Build history of the part. All positions in model axes, mm. Face numbers are marked on the shaded views. A direction names the side the tool comes from. Round coordinates to 2 decimals unless told otherwise and drop trailing zeros. Loops run counter-clockwise (first coordinate to the right, second up) from the corner with the lowest first, then second, coordinate; pieces in that order, holes last. Notation, with made-up numbers: M -35,26.5 L 20,26.5 A19 ccw 20,47.5 Z; hole C 51.5,16.25 d4. An arc over 180 degrees is marked long. Write each question's results on one line, items separated by ' | '. Start each with the question number.
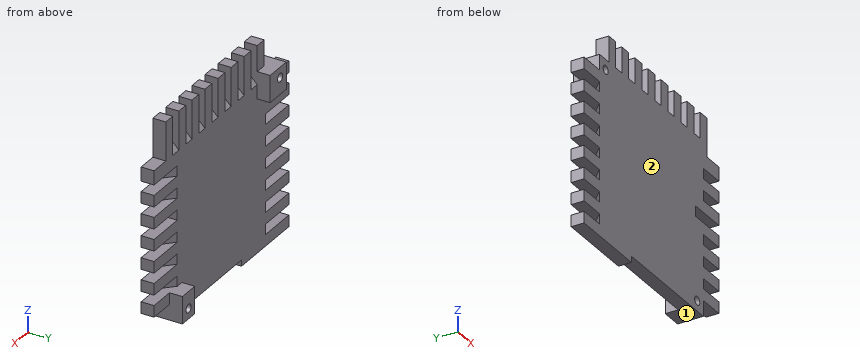
```python
from build123d import *

# Parameters (mm, degrees)
BASE_OUTLINE_R      = 0.5
BOSS_EXTRUDE1_DEPTH = 1.5
DRAFT2_ANGLE        = 45
SPACER_OUTLINE_W    = 3.14
SPACER_OUTLINE_H    = 3.14
SPACER_OUTLINE_W_2  = 2.4
SPACER_OUTLINE_H_2  = 3.16
BOSS_EXTRUDE2_DEPTH = 1.5
SKETCH1_3_R         = 0.5
CUT_EXTRUDE1_DEPTH  = 5.5


with BuildPart() as part:
    # Base outline → Boss-Extrude1 (new body)
    with BuildSketch(Plane(origin=(0, 0, 0), x_dir=(1, 0, 0), z_dir=(0, 1, 0))):
        Polygon((6.201628494, 20.2), (20.2, 20.2), (20.2, 18.38), (23.2, 18.38), (23.2, 17.04), (20.2, 17.04), (18.7, 17.04), (18.7, 15.84), (20.2, 15.84), (23.2, 15.84), (23.2, 14.5), (20.2, 14.5), (18.7, 14.5), (18.7, 13.3), (20.2, 13.3), (23.2, 13.3), (23.2, 11.96), (20.2, 11.96), (18.7, 11.96), (18.7, 10.76), (20.2, 10.76), (23.2, 10.76), (23.2, 9.42), (20.2, 9.42), (18.7, 9.42), (18.7, 8.22), (20.2, 8.22), (23.2, 8.22), (23.2, 6.88), (20.2, 6.88), (18.7, 6.88), (18.7, 5.68), (20.2, 5.68), (23.2, 5.68), (23.2, 4.34), (20.2, 4.34), (18.7, 4.34), (18.7, 3.14), (20.2, 3.14), (23.2, 3.14), (23.2, 1.5), (20.92, 1.5), (20.92, -3), (19.58, -3), (19.58, 0), (19.58, 1.5), (18.38, 1.5), (18.38, 0), (18.38, -3), (17.04, -3), (17.04, 0), (17.04, 1.5), (15.84, 1.5), (15.84, 0), (15.84, -3), (14.5, -3), (14.5, 0), (14.5, 1.5), (13.3, 1.5), (13.3, 0), (13.3, -3), (11.96, -3), (11.96, 0), (11.96, 1.5), (10.76, 1.5), (10.76, 0), (10.76, -3), (9.42, -3), (9.42, 0), (9.42, 1.5), (8.22, 1.5), (8.22, 0), (8.22, -3), (6.88, -3), (6.88, 0), (6.88, 1.5), (5.68, 1.5), (5.68, 0), (5.68, -3), (4.34, -3), (4.34, 0), (4.34, 1.5), (3.14, 1.5), (3.14, 0), (3.14, -3), (1.8, -3), (1.8, 0), (0, 0), (0, 1.8), (-3, 1.8), (-3, 3.14), (0, 3.14), (1.5, 3.14), (1.5, 4.34), (0, 4.34), (-3, 4.34), (-3, 5.68), (0, 5.68), (1.5, 5.68), (1.5, 6.88), (0, 6.88), (-3, 6.88), (-3, 8.22), (0, 8.22), (1.5, 8.22), (1.5, 9.42), (0, 9.42), (-3, 9.42), (-3, 10.76), (0, 10.76), (1.5, 10.76), (1.5, 11.96), (0, 11.96), (-3, 11.96), (-3, 13.3), (0, 13.3), (1.5, 13.3), (1.5, 14.5), (0, 14.5), (-3, 14.5), (-3, 15.84), (0, 15.84), (1.5, 15.84), (1.5, 17.04), (0, 17.04), (-3, 17.04), (-3, 18.38), (0, 18.38), (1.5, 18.38), (1.5, 19.58), (0, 19.58), (-3, 19.58), (-3, 20.92), (6.201628494, 20.92), align=None)
        with Locations(Location((1.2, 1.2, 0), (0, 0, 270))):
            Circle(BASE_OUTLINE_R, mode=Mode.SUBTRACT)
        with Locations(Location((19, 19, 0), (0, 0, 270))):
            Circle(BASE_OUTLINE_R, mode=Mode.SUBTRACT)
    extrude(amount=BOSS_EXTRUDE1_DEPTH)

    # Draft2
    draft2_faces = [part.faces().sort_by_distance(p)[0] for p in [
        (1.5, 0.75, -18.98),
        (1.5, 0.75, -16.44),
        (1.5, 0.75, -13.9),
        (1.5, 0.75, -11.36),
        (1.5, 0.75, -8.82),
        (1.5, 0.75, -6.28),
        (1.5, 0.75, -3.74),
        (18.7, 0.75, -16.44),
        (18.7, 0.75, -13.9),
        (18.7, 0.75, -11.36),
        (18.7, 0.75, -6.28),
        (18.7, 0.75, -3.74),
        (18.98, 0.75, -1.5),
        (16.44, 0.75, -1.5),
        (13.9, 0.75, -1.5),
        (11.36, 0.75, -1.5),
        (8.82, 0.75, -1.5),
        (6.28, 0.75, -1.5),
        (3.74, 0.75, -1.5),
    ]]
    draft(draft2_faces, Plane.ZX.offset(1.5), DRAFT2_ANGLE)

    # Spacer outline → Boss-Extrude2 (add)
    with BuildSketch(Plane(origin=(0, 1.5, 0), x_dir=(1, 0, 0), z_dir=(0, 1, 0))):
        with Locations((1.57, 1.57)):
            Rectangle(SPACER_OUTLINE_W, SPACER_OUTLINE_H)
        with Locations((19, 18.62)):
            Rectangle(SPACER_OUTLINE_W_2, SPACER_OUTLINE_H_2)
    extrude(amount=BOSS_EXTRUDE2_DEPTH)

    # Sketch1_3 → Cut-Extrude1 (cut)
    with BuildSketch(Plane(origin=(0, 0, 0), x_dir=(1, 0, 0), z_dir=(0, 1, 0))):
        with Locations(Location((1.2, 1.2, 0), (0, 0, 270))):
            Circle(SKETCH1_3_R)
        with Locations(Location((19, 19, 0), (0, 0, 90))):
            Circle(SKETCH1_3_R)
    extrude(amount=CUT_EXTRUDE1_DEPTH, mode=Mode.SUBTRACT)


solid = part.part
```
Item 1: Drill centre lines: line 1 along Z through (x, y) = (19, 2.15); line 2 along X through (y, z) = (1.7, -1.2); line 3 along X through (y, z) = (1.75, -19). Where is each one in solid material? Low to high. Write a range as [from, to].
Item 2: Tool access for the marked faces 1 and 2: list every direction of +Z, -Z, +X, -X, +Y, -Y with a clear straight run to the whole face (end or side of a thin tool).
Item 3: Saw through at B-B, the plane x = 19. State how many separate pieces and enclosed holes the cut face has, then the cut area to 3 significant figures.
Item 4: Saw through at C-C, the plane z = -19. Give the cut face in (x, y).
Item 5: Drop flat-ended pins along their axis: pin 1 (1.6 mm diameter, centred on y = 1, z = 0.5, fed in from +X); pin 2 (1.2 mm diameter, centred on x = -0.5, y = 1, fed in from +Z); pin 3 (1.2 mm diameter, centred on y = 1, z = 1, fed in from -X). Give the stop position or say it passes through.
Item 6: Saw through at D-D, the plane z = -4.75. Give the cut face in (x, y).
Item 7: Saw through at A-A, the plane y = 2.55. Give the cut face in (x, z), then the cut area to 3 significant figures.
Working result:
1) line 1: z = [-20.2, -19.5], [-18.5, -17.04] | line 2: x = [0, 0.7], [1.7, 3.14] | line 3: x = [17.8, 18.5], [19.5, 20.2]
2) face 1: -Z, +X, +Y, -Y | face 2: +Z, -Z, +X, -X, -Y
3) separate pieces: 3 | enclosed holes: 0 | area: 27.3 mm²
4) outline: M 0,0 L 18.5,0 L 18.5,3 L 17.8,3 L 17.8,1.5 L 1.5,1.5 Z; M 19.5,0 L 20.2,0 L 20.2,3 L 19.5,3 Z
5) pin 1: stops at x = 20.92 | pin 2: stops at z = 0 | pin 3: stops at x = 1.8
6) outline: M -3,0 L 23.2,0 L 23.2,1.5 L -3,1.5 Z
7) outline: M 0,-3.14 L 3.14,-3.14 L 3.14,0 L 0,0 Z; M 17.8,-20.2 L 20.2,-20.2 L 20.2,-17.04 L 17.8,-17.04 Z; hole C 1.2,-1.2 d1; hole C 19,-19 d1 | area: 15.9 mm²
